Could you check a few things on this model? Use its own coordinates, in mm. Coordinates: 2 decimals unless noted, no trailing zeros. Loops run counter-clockwise (first coordinate to the right, second up) from the corner with the lowest first, then second, coordinate; pieces in that order, holes last.
from build123d import *

# Parameters (mm, degrees)
SKETCH1_R           = 48.26
SKETCH1_R_2         = 11.375
BOSS_EXTRUDE1_DEPTH = 7.62
SKETCH3_R           = 1.7145
CUT_EXTRUDE1_DEPTH  = 3.81
SKETCH5_R           = 48.26
SKETCH5_R_2         = 40.64
BOSS_EXTRUDE2_DEPTH = 17.78
SKETCH10_R          = 2.794
CUT_EXTRUDE2_DEPTH  = 3.556
SKETCH11_R          = 2.000000064
CUT_EXTRUDE3_DEPTH  = 100.757829768
SKETCH13_R          = 29.591
SKETCH13_R_2        = 26.289
CUT_EXTRUDE7_DEPTH  = 3.81


with BuildPart() as part:
    # Sketch1 → Boss-Extrude1 (new body)
    with BuildSketch(Plane.XY):
        with Locations(Location((21.15, -21.15, 0), (0, 0, 180))):
            Circle(SKETCH1_R)
        with Locations(Location((21.15, -21.15, 0), (0, 0, 180))):
            Circle(SKETCH1_R_2, mode=Mode.SUBTRACT)
    extrude(amount=BOSS_EXTRUDE1_DEPTH)

    # Sketch3 → Cut-Extrude1 (cut)
    with BuildSketch(Plane.XY.offset(7.62)):
        with Locations((21.15, 16.315)):
            Circle(SKETCH3_R)
        with Locations((30.115961363, 15.22633519)):
            Circle(SKETCH3_R)
        with Locations((38.560853641, 12.023610001)):
            Circle(SKETCH3_R)
        with Locations((45.993890391, 6.89295518)):
            Circle(SKETCH3_R)
        with Locations((51.983090536, 0.132545736)):
            Circle(SKETCH3_R)
        with Locations((56.180383532, -7.864727907)):
            Circle(SKETCH3_R)
        with Locations((58.341837968, -16.634093274)):
            Circle(SKETCH3_R)
        with Locations((58.341837968, -25.665906726)):
            Circle(SKETCH3_R)
        with Locations((56.180383532, -34.435272093)):
            Circle(SKETCH3_R)
        with Locations((51.983090536, -42.432545736)):
            Circle(SKETCH3_R)
        with Locations((45.993890391, -49.19295518)):
            Circle(SKETCH3_R)
        with Locations((38.560853641, -54.323610001)):
            Circle(SKETCH3_R)
        with Locations((30.115961363, -57.52633519)):
            Circle(SKETCH3_R)
        with Locations((21.15, -58.615)):
            Circle(SKETCH3_R)
        with Locations((12.184038637, -57.52633519)):
            Circle(SKETCH3_R)
        with Locations((3.739146359, -54.323610001)):
            Circle(SKETCH3_R)
        with Locations((-3.693890391, -49.19295518)):
            Circle(SKETCH3_R)
        with Locations((-9.683090536, -42.432545736)):
            Circle(SKETCH3_R)
        with Locations((-13.880383532, -34.435272093)):
            Circle(SKETCH3_R)
        with Locations((-16.041837968, -25.665906726)):
            Circle(SKETCH3_R)
        with Locations((-16.041837968, -16.634093274)):
            Circle(SKETCH3_R)
        with Locations((-13.880383532, -7.864727907)):
            Circle(SKETCH3_R)
        with Locations((-9.683090536, 0.132545736)):
            Circle(SKETCH3_R)
        with Locations((-3.693890391, 6.89295518)):
            Circle(SKETCH3_R)
        with Locations((3.739146359, 12.023610001)):
            Circle(SKETCH3_R)
        with Locations((12.184038637, 15.22633519)):
            Circle(SKETCH3_R)
    extrude(amount=-CUT_EXTRUDE1_DEPTH, mode=Mode.SUBTRACT)

    # Sketch5 → Boss-Extrude2 (add)
    with BuildSketch(Plane.XY.offset(7.62)):
        with Locations(Location((21.15, -21.15, 0), (0, 0, 180))):
            Circle(SKETCH5_R)
        with Locations((21.15, -21.15)):
            Circle(SKETCH5_R_2, mode=Mode.SUBTRACT)
    extrude(amount=BOSS_EXTRUDE2_DEPTH)

    # Sketch10 → Cut-Extrude2 (cut)
    with BuildSketch(Plane.XY.offset(7.62)):
        with Locations((36.65, -36.65)):
            Circle(SKETCH10_R)
        with Locations((5.65, -36.65)):
            Circle(SKETCH10_R)
        with Locations((5.65, -5.65)):
            Circle(SKETCH10_R)
        with Locations((36.65, -5.65)):
            Circle(SKETCH10_R)
    extrude(amount=-CUT_EXTRUDE2_DEPTH, mode=Mode.SUBTRACT)

    # Sketch11 → Cut-Extrude3 (cut, through all)
    with BuildSketch(Plane.XY.offset(7.62)):
        with Locations((36.65, -36.65)):
            Circle(SKETCH11_R)
        with Locations((5.65, -36.65)):
            Circle(SKETCH11_R)
        with Locations((36.65, -5.65)):
            Circle(SKETCH11_R)
        with Locations((5.65, -5.65)):
            Circle(SKETCH11_R)
    extrude(amount=-CUT_EXTRUDE3_DEPTH, mode=Mode.SUBTRACT)

    # Sketch13 → Cut-Extrude7 (cut)
    with BuildSketch(Plane(origin=(0, 0, 7.62), x_dir=(-1, 0, 0), z_dir=(0, 0, -1))):
        with Locations(Location((-21.15, -21.15, 0), (0, 0, 180))):
            Circle(SKETCH13_R)
        with Locations(Location((-21.15, -21.15, 0), (0, 0, 180))):
            Circle(SKETCH13_R_2, mode=Mode.SUBTRACT)
    extrude(amount=CUT_EXTRUDE7_DEPTH, mode=Mode.SUBTRACT)


solid = part.part
(1) Imagine slicing it at B-B, the plane z = 6.5. State how many separate pieces and enclosed holes the cut face has, and give its area (3 significant figures).
Answers:
separate pieces: 2
enclosed holes: 32
area: 5,990 mm2
(2) Imagine slicing it at C-C, the plane z = 21. Write out the boundary of the cut face in (x, y), and give its area (3 significant figures).
Answers:
outline: circle Ø96.52 at (21.15, -21.15); hole circle Ø81.28 at (21.15, -21.15)
area: 2,130 mm2
(3) Imagine slicing it at A-A, the plane y = -21.15. Write out the boundary of the cut face in (x, z) (3 decimals), and give its area (3 significant figures).
Answers:
outline: (-27.11, 0) - (9.775, 0) - (9.775, 7.62) - (-5.139, 7.62) - (-5.139, 3.81) - (-8.441, 3.81) - (-8.441, 7.62) - (-19.49, 7.62) - (-19.49, 25.4) - (-27.11, 25.4) - close; (32.525, 0) - (69.41, 0) - (69.41, 25.4) - (61.79, 25.4) - (61.79, 7.62) - (50.741, 7.62) - (50.741, 3.81) - (47.439, 3.81) - (47.439, 7.62) - (32.525, 7.62) - close
area: 808 mm2
(4) I need wall thicknesses on probe 1 along X at (y, z) = (-5, 5.25); probe 2 along Z at (x, y) = (53, -10); probe 3 along Y at (x, z) = (-8.5, 1.5). Which ranges of each line are inside material? Lowest first, please.
Answers:
probe 1: x = -24.33 to -3.65, 0.41 to 2.93, 8.37 to 33.93, 39.37 to 41.89, 45.95 to 66.63
probe 2: z = 0 to 7.62
probe 3: y = -59.23 to 16.93
(5) For pin 1 (1.5 mm diameter, centred on x = -10, y = -59.5, fed in from -Z) (3 decimals); pin 2 (4 mm diameter, centred on y = 1, z = 15.5, fed in from -X); pin 3 (6.5 mm diameter, centred on x = 36.65, y = -5.65, fed in from +Z); pin 4 (2 mm diameter, centred on x = 30.12, y = 15.23, fed in from +Z), each with a flat end and sliding along its axis, tell me the tip position at first contact or that it passes through.
Answers:
pin 1: passes through
pin 2: stops at x = -22.7
pin 3: stops at z = 7.62
pin 4: stops at z = 3.81
